```python
from build123d import *

# Parameters (mm, degrees)
SKETCH2_W               = 50
SKETCH2_H               = 130
BOSS_EXTRUDE2_DEPTH     = 8
CUT_EXTRUDE1_DEPTH      = 20
CUT_EXTRUDE1_DEPTH_BACK = 20
SKETCH4_R               = 11
SKETCH7_W               = 30
SKETCH7_H               = 25
BOSS_EXTRUDE3_DEPTH     = 50
SKETCH8_R               = 6.223
CUT_EXTRUDE2_DEPTH      = 50


with BuildPart() as part:
    # Sketch2 → Boss-Extrude2 (new body)
    with BuildSketch(Plane(origin=(0, 0, 0), x_dir=(0, 0, -1), z_dir=(1, 0, 0))):
        with Locations((25, 65)):
            Rectangle(SKETCH2_W, SKETCH2_H)
    extrude(amount=BOSS_EXTRUDE2_DEPTH)

    # Sketch4 → Cut-Extrude1 (cut, two sides: drawn at the far end of the back side and taken through both)
    with BuildSketch(Plane(origin=(0, 0, 0), x_dir=(0, 0, -1), z_dir=(1, 0, 0)).offset(-CUT_EXTRUDE1_DEPTH_BACK)):
        with Locations(Location((25, 15, 0), (0, 0, 180))):
            Circle(SKETCH4_R)
    extrude(amount=CUT_EXTRUDE1_DEPTH + CUT_EXTRUDE1_DEPTH_BACK, mode=Mode.SUBTRACT)

    # Sketch7 → Boss-Extrude3 (add)
    with BuildSketch(Plane(origin=(8, 0, 0), x_dir=(0, 0, -1), z_dir=(1, 0, 0))):
        with Locations((25, 15)):
            Rectangle(SKETCH7_W, SKETCH7_H)
    extrude(amount=BOSS_EXTRUDE3_DEPTH)

    # Sketch8 → Cut-Extrude2 (cut)
    with BuildSketch(Plane(origin=(58, 0, 0), x_dir=(0, 0, -1), z_dir=(1, 0, 0))):
        with Locations((25, 15)):
            Circle(SKETCH8_R)
    extrude(amount=-CUT_EXTRUDE2_DEPTH, mode=Mode.SUBTRACT)


solid = part.part
```
Geometry: final body of the model. Coordinates: model frame, mm. A direction names the side the tool comes from. Round coordinates to 2 decimals unless told otherwise and drop trailing zeros. Order: outer loops, then holes, each group sorted by start corner. A loop starts at its lowest first (then second) coordinate and runs counter-clockwise, first axis right, second up. Notation, with made-up numbers: (-29.5, -38) -> (-18.5, -38) arc R30 ccw to (-18.5, -3) -> close; hole circle Ø9 at (22, 40). An arc over 180 degrees is marked (long way). Use one line per item in the form item = value.
(1) Ray query, probe 1 along Y at (x, z) = (19, -25); probe 2 along Y at (x, z) = (14, -11); probe 3 along Z at (x, y) = (28, 25.5). Return the intervals inside material, ascending. Write a range as [from, to].
Results list:
probe_1 = [2.5, 8.78], [21.22, 27.5]
probe_2 = [2.5, 27.5]
probe_3 = [-40, -10]
(2) Section A-A on z = -25. Return loops of the section in (x, y).
Results list:
outline = (0, 0) -> (8, 0) -> (8, 2.5) -> (58, 2.5) -> (58, 8.78) -> (8, 8.78) -> (8, 4) -> (0, 4) -> close; (0, 26) -> (8, 26) -> (8, 21.22) -> (58, 21.22) -> (58, 27.5) -> (8, 27.5) -> (8, 130) -> (0, 130) -> close
(3) Access query for faces 4 (the face through (33, 2.5, -25)), 5 (the face through (33, 27.5, -25)), 6 (the face through (33, 15, -10)), 7 (the face through (3.944, 24.759, -19.924)). Directions: +Z, -Z, +X, -X, +Y, -Y. A direction counts if a zero-diameter tool reaches every point of the face in a straight line with its end or side. Return the directions, or none.
Results list:
face_4 = +Z, -Z, +X, -Y
face_5 = +Z, -Z, +X, +Y
face_6 = +Z, +X, +Y, -Y
face_7 = -X
(4) Section B-B on y = 15. Return loops of the section in (x, z).
Results list:
outline = (0, -50) -> (8, -50) -> (8, -40) -> (58, -40) -> (58, -31.22) -> (8, -31.22) -> (8, -36) -> (0, -36) -> close; (0, -14) -> (8, -14) -> (8, -18.78) -> (58, -18.78) -> (58, -10) -> (8, -10) -> (8, 0) -> (0, 0) -> close
(5) Section C-C on x = 32.5. Return loops of the section in (y, z).
Results list:
outline = (2.5, -40) -> (27.5, -40) -> (27.5, -10) -> (2.5, -10) -> close; hole circle Ø12.45 at (15, -25)
(6) First-contact query: pin 1 Ø3 at (x, z) = (49, -35.5) entering from -Y; pin 2 Ø15 at (y, z) = (86.5, -24.5) entering from +X; pin 3 Ø10 at (x, z) = (29.5, -21.5) entering from +Y. Flat tips, straight axial feed; report the tip coordinate or a pass-through.
Results list:
pin_1 = 2.5
pin_2 = 8
pin_3 = 27.5
(7) Draft query along Z for faces 1 (the face through (8, 10, -30)), 2 (the face through (4, 64, 0)), 3 (the face through (33, 15, -40)). Return one class per face: pulls with the +Z half, pulls with the -Z half, needs draft (parallel to the pull), parting line crosses it, or undercut.
Results list:
face_1 = undercut
face_2 = pulls with the +Z half
face_3 = pulls with the -Z half
(8) Section D-D on y = 84. Return loops of the section in (x, z), and give its area (3 significant figures).
Results list:
outline = (0, -50) -> (8, -50) -> (8, 0) -> (0, 0) -> close
area = 400 mm^2
